```python
from build123d import *

# Parameters (mm, degrees)
F0_R     = 11
F0_R_2   = 5.75
F0_R_3   = 4
F0_R_4   = 3
F1_DEPTH = 2
F2_DEPTH = 3
F3_DEPTH = 6
F4_R     = 0.5


with BuildPart() as f1:
    # F0 (on Top) → F1 (new body)
    with BuildSketch(Plane.XY):
        Circle(F0_R)
        Circle(F0_R_2, mode=Mode.SUBTRACT)
        Circle(F0_R_2)
        Circle(F0_R_3, mode=Mode.SUBTRACT)
        Circle(F0_R_3)
        Circle(F0_R_4, mode=Mode.SUBTRACT)
        Circle(F0_R_4)
    extrude(amount=F1_DEPTH)

    # F0 (on Top) → F2 (join)
    with BuildSketch(Plane.XY):
        Circle(F0_R_2)
        Circle(F0_R_3, mode=Mode.SUBTRACT)
    extrude(amount=F2_DEPTH)

    # F0 (on Top) → F3 (join)
    with BuildSketch(Plane.XY):
        Circle(F0_R_3)
        Circle(F0_R_4, mode=Mode.SUBTRACT)
    extrude(amount=F3_DEPTH)

    # F4
    f4_edges = [f1.edges().sort_by_distance(p)[0] for p in [
        (-4, 0, 6),
        (-5.75, 0, 3),
        (-11, 0, 2),
        (-11, 0, 0),
    ]]
    fillet(f4_edges, radius=F4_R)


solid = f1.part
```
Verification items for the finished model (mm, model axes). A direction names the side the tool comes from. Give positions to 0.01 mm unless a question says otherwise; leave off trailing zeros. Loops run counter-clockwise (first coordinate to the right, second up) from the corner with the lowest first, then second, coordinate; pieces in that order, holes last.
1. Section check A-A, the plane x = 0. Enter the section's corners in (y, z).
2. Mould release check, pull along Y, two halves, no side actions. Record for faces 1 (the cylindrical face through (-0.75, 5.7, 2.25)), 2 (the cylindrical face through (-3, 0, 4)), 3 (the flat face through (3, 1, 6)): released by +Y, released by -Y, zero draft, split by the parting line, or undercut.
3. Thickness scan on line 1 (Y direction, x = 0, z = 4.85); line 2 (Z direction, x = 4.5, y = -8.25); line 3 (Y direction, x = 0.25, z = 1.15). Record the ranges inside material, lowest first.
4. Set-up check for faces 4 (the cylindrical face through (-2.38, -10.74, 0.99)), 5 (the flat face through (-4, -2, 3)): record each of +Z, -Z, +X, -X, +Y, -Y from which the full face is reachable in a straight line by a thin tool's end or side.
5. Section check B-B, the plane z = 3.5. Enter the section's corners in (x, y), then the cut area to 3 significant figures.
6. Go/stop test with flat-tipped pins: pin 1 Ø3 at (x, z) = (5.5, 3) entering from -Y; pin 2 Ø1 at (x, y) = (0.5, 1.5) entering from +Z; pin 3 Ø3 at (x, z) = (-7.5, 2) entering from +Y. Record where each tip stops, or that it passes through.
Geometry says:
1. outline: (-11, 0.5) arc R0.5 ccw to (-10.5, 0) - (10.5, 0) arc R0.5 ccw to (11, 0.5) - (11, 1.5) arc R0.5 ccw to (10.5, 2) - (5.75, 2) - (5.75, 2.5) arc R0.5 ccw to (5.25, 3) - (4, 3) - (4, 5.5) arc R0.5 ccw to (3.5, 6) - (3, 6) - (3, 2) - (-3, 2) - (-3, 6) - (-3.5, 6) arc R0.5 ccw to (-4, 5.5) - (-4, 3) - (-5.25, 3) arc R0.5 ccw to (-5.75, 2.5) - (-5.75, 2) - (-10.5, 2) arc R0.5 ccw to (-11, 1.5) - close
2. face 1: split by the parting line
2. face 2: undercut
2. face 3: zero draft
3. line 1: y = -4 to -3, 3 to 4
3. line 2: z = 0 to 2
3. line 3: y = -11 to 11
4. face 4: +Z, -Z
4. face 5: +Z
5. outline: circle Ø8 at (0, 0); hole circle Ø6 at (0, 0)
5. area: 22.0 mm2
6. pin 1: stops at y = -9.89
6. pin 2: stops at z = 2
6. pin 3: stops at y = 9.17
